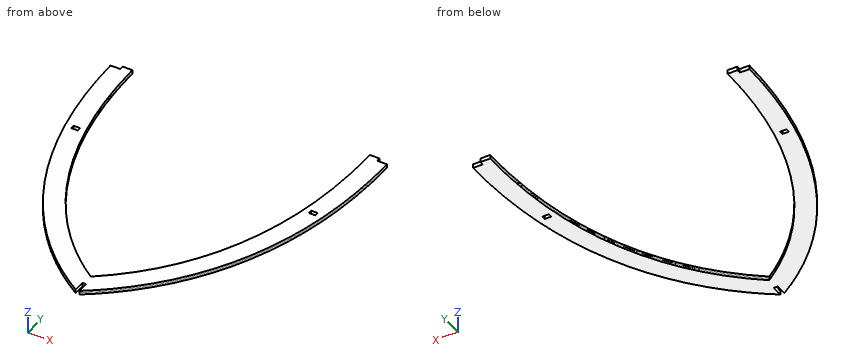
```python
from build123d import *

# Parameters (mm, degrees)
SKETCH1_W           = 5
SKETCH1_H           = 3
BOSS_EXTRUDE1_DEPTH = 1.5
SKETCH2_W           = 3
SKETCH2_H           = 9.494035225
CUT_EXTRUDE1_DEPTH  = 3


with BuildPart() as part:
    # Sketch1 → Boss-Extrude1 (new body, symmetric)
    with BuildSketch(Plane.XY):
        with BuildLine():
            Line((-106, -83), (-98.5, -83))
            Line((-98.5, -83), (-98.5, -80))
            Line((-98.5, -80), (-91, -80))
            Line((-91, -80), (-91, -83))
            add(Edge.make_bspline(
                [(-91, -83), (-91, -88.068550738), (-90.784224976, -98.220481237), (-89.47168793, -118.377767283), (-86.146815138, -143.230800288), (-79.368059247, -172.071120857), (-69.71738881, -199.531988744), (-57.11831244, -225.231718508), (-44.09611353, -244.888891231), (-32.112008882, -259.401886537), (-22.324804426, -269.642683196), (-13.481107719, -277.613388782), (-5.992695326, -283.625797901), (-2.089373231, -286.521065709), (-0.116739636, -287.926353347)],
                knots=[0, 0, 0, 0, 0.059983469, 0.119966937, 0.239933875, 0.359900812, 0.47986775, 0.599834687, 0.719801625, 0.779785093, 0.839768562, 0.899752031, 0.929743765, 0.9597355, 0.9597355, 0.9597355, 0.9597355], degree=3))
            add(Edge.make_bspline(
                [(-0.116739636, -287.926353347), (1.870810321, -286.480217138), (5.811438827, -283.506382084), (13.355962702, -277.384642576), (22.257609381, -269.345287034), (32.090104581, -259.121737951), (44.109675826, -244.741072781), (57.139620096, -225.411627313), (69.725154077, -200.204558319), (79.363006417, -173.160517049), (85.009288933, -149.261906753), (88.135960803, -129.439309105), (89.796426225, -114.252560891), (90.618872692, -101.350995082), (90.945843548, -90.910045133), (91, -85.632026579), (91, -83)],
                knots=[0, 0, 0, 0, 0.030008035, 0.060016069, 0.120032138, 0.180048207, 0.240064276, 0.360096414, 0.480128553, 0.600160691, 0.720192829, 0.780208898, 0.840224967, 0.900241036, 0.930249071, 0.960257105, 0.960257105, 0.960257105, 0.960257105], degree=3))
            Line((91, -83), (91, -80))
            Line((91, -80), (98.5, -80))
            Line((98.5, -80), (98.5, -83))
            Line((98.5, -83), (106, -83))
            add(Edge.make_bspline(
                [(106, -83), (106, -174.443319162), (74.762940933, -256.782973383), (0, -306.089272366)],
                knots=[0, 0, 0, 0, 1, 1, 1, 1], degree=3))
            add(Edge.make_bspline(
                [(-106, -83), (-106, -171.171703536), (-74.762940933, -258.439171974), (0, -306.089272366)],
                knots=[0, 0, 0, 0, 1, 1, 1, 1], degree=3))
        make_face()
        with Locations((-91.1, -153.5)):
            Rectangle(SKETCH1_W, SKETCH1_H, mode=Mode.SUBTRACT)
        with Locations((91.1, -153.5)):
            Rectangle(SKETCH1_W, SKETCH1_H, mode=Mode.SUBTRACT)
    extrude(amount=BOSS_EXTRUDE1_DEPTH, both=True)

    # Sketch2 → Cut-Extrude1 (cut)
    with BuildSketch(Plane.XY.offset(1.5)):
        with Locations((0, -301.342254754)):
            Rectangle(SKETCH2_W, SKETCH2_H)
    extrude(amount=-CUT_EXTRUDE1_DEPTH, mode=Mode.SUBTRACT)


solid = part.part
```
Design review of the part built by this model. Coordinates are the model's own, in mm. Coordinates: 2 decimals unless noted, no trailing zeros. One line per item, written item: value. Start each with the question number.
Q1. Take a section at A-A, the plane z = 0.9. Give the number of separate pieces and of enclosed holes in the cut face, then the cut area to 3 significant figures.
Q2. Insertion check: pin 1 Ø0.9 at (y, z) = (-300.5, 0) entering from +X; pin 2 Ø1.5 at (y, z) = (-81.5, 0) entering from +X; pin 3 Ø1.5 at (y, z) = (-154, 0) entering from +X. Each pin has a flat end and moves straight along its axis. Give the tip position at first contact, or say it passes through.
Q3. For probe 1 along X at (y, z) = (-174.5, 1); probe 2 along X at (y, z) = (-89, 0.3); probe 3 along Y at (x, z) = (26, 1.3), list the stretches that pass through material, from the lowest coordinate up.
Values follow:
1. separate pieces: 1
1. enclosed holes: 2
1. area: 7,350 mm2
2. pin 1: stops at x = 8.72
2. pin 2: stops at x = 98.5
2. pin 3: stops at x = 99.21
3. probe 1: x = -93.73 to -78.1, 78.41 to 94.03
3. probe 2: x = -105.95 to -90.95, 90.95 to 105.95
3. probe 3: y = -286.12 to -265.38
